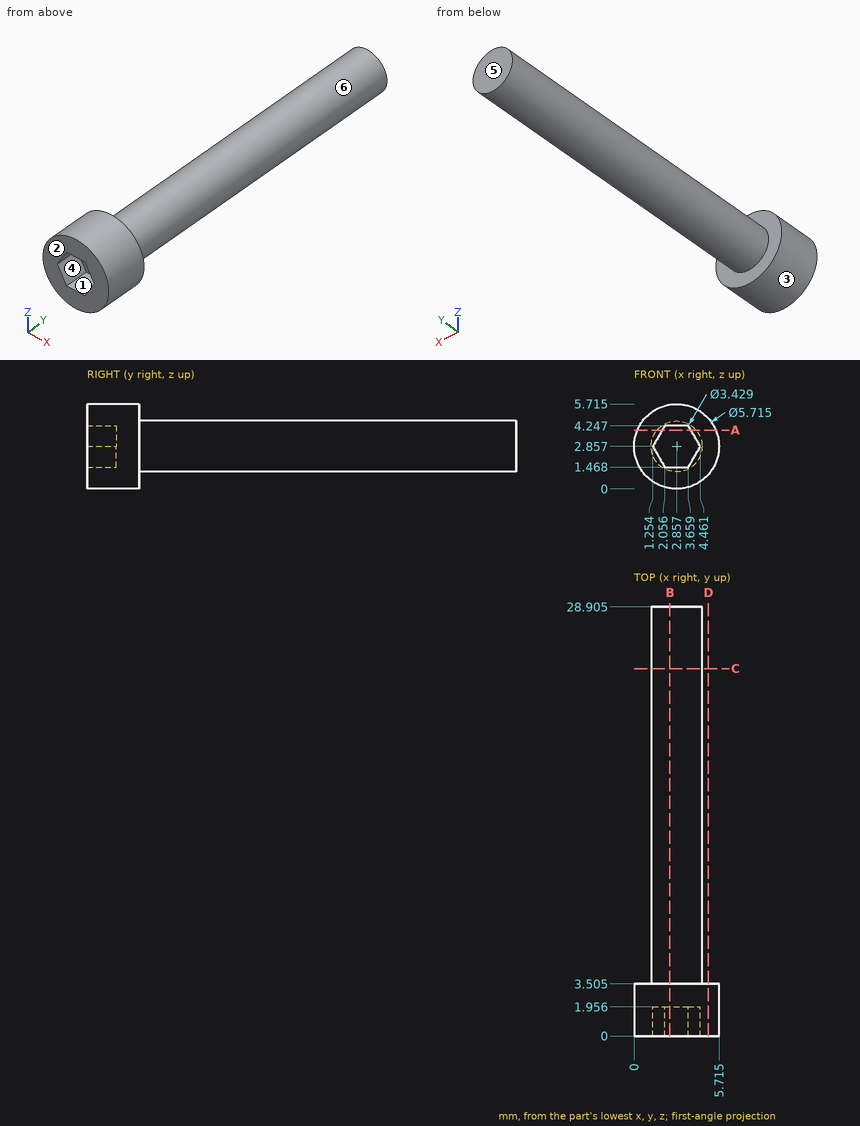
The drawing under review shows one solid part. Ordinate dimensions are in mm from its lowest x, y, z. A direction names the side the tool comes from. Coordinates: 2 decimals unless noted, no trailing zeros. Loops run counter-clockwise (first coordinate to the right, second up) from the corner with the lowest first, then second, coordinate; pieces in that order, holes last. Notation, with made-up numbers: (-9.75, 42.5) -> (39.25, 42.5) arc R24 cw to (39.25, 74.5) -> close; hole circle Ø7 at (28.5, 35.25). An arc over 180 degrees is marked (long way). Answer as a JSON object with one key per item and string values.
Q1. Take a section at D-D on x = 5. Give the boundary of the cut face in (y, z) (1 decimal).
Answer block:
{"outline": "(0, 1) -> (3.5, 1) -> (3.5, 4.7) -> (0, 4.7) -> close"}
Q2. To check wall thickness, follow L1, parallel to X at y = 16, z = 2.8 (1 decimal); L2, parallel to Y at x = 3.5, z = 2.35 (1 decimal). State the ranges of each line that lie inside material, in increasing order.
Answer block:
{"L1": "x = 1.1 to 4.6", "L2": "y = 2 to 28.9"}
Q3. Take a section at C-C on y = 24.75. Give the boundary of the cut face in (x, z) (1 decimal).
Answer block:
{"outline": "circle Ø3.4 at (2.9, 2.9)"}
Q4. The part is to be moulded in two halves that separate along X. For the marked faces 1, 2, 3 and 4, say which applies: +X half, -X half, draft (parallel to the pull), parting line (faces both ways), or undercut.
Answer block:
{"face 1": "undercut", "face 2": "draft", "face 3": "parting line", "face 4": "undercut"}
Q5. Take a section at B-B on x = 2.4. Give the boundary of the cut face in (y, z) (1 decimal).
Answer block:
{"outline": "(0, 0) -> (3.5, 0) -> (3.5, 1.2) -> (28.9, 1.2) -> (28.9, 4.5) -> (3.5, 4.5) -> (3.5, 5.7) -> (0, 5.7) -> (0, 4.2) -> (2, 4.2) -> (2, 1.5) -> (0, 1.5) -> close"}
Q6. Tool access review of the marked faces 5 and 6: name each direction out of +Z, -Z, +X, -X, +Y, -Y from which nothing blocks a thin tool from reaching the whole face with its end or side.
Answer block:
{"face 5": "+Z, -Z, +X, -X, +Y", "face 6": "+Y"}
Q7. Clearance check with flat-ended pins moving along their axes: pin 1 Ø1 at (x, y) = (3, 24) entering from -Z; pin 2 Ø1.5 at (y, z) = (20.5, 4.5) entering from -X (1 decimal); pin 3 Ø2 at (y, z) = (16.5, 2.5) entering from -X. State where each tip first meets the part, or that it passes through.
Answer block:
{"pin 1": "stops at z = 1.14", "pin 2": "stops at x = 1.4", "pin 3": "stops at x = 1.14"}
Q8. Take a section at A-A on z = 3.95. Give the boundary of the cut face in (x, y) (1 decimal).
Answer block:
{"outline": "(0.2, 0) -> (1.9, 0) -> (1.9, 2) -> (3.8, 2) -> (3.8, 0) -> (5.5, 0) -> (5.5, 3.5) -> (4.2, 3.5) -> (4.2, 28.9) -> (1.5, 28.9) -> (1.5, 3.5) -> (0.2, 3.5) -> close"}
